Source: CAD feature listing. Evaluate the final solid. Frame: model axes, mm. A direction names the side the tool comes from. Coordinates: 2 decimals unless noted, no trailing zeros. Loops run counter-clockwise (first coordinate to the right, second up) from the corner with the lowest first, then second, coordinate; pieces in that order, holes last. Notation, with made-up numbers: (-12, 2) - (-5, 2) arc R21 ccw to (-5, 16) - close; hole circle Ø8 at (27.5, 67.25). An arc over 180 degrees is marked (long way). Use CSV: the item, a comma, the result in double quotes. Start each with the question number.
Autodesk Inventor part; units mm, degrees
ref_plane "YZ Plane" through (0, 0, 0) normal (1, 0, 0) x (0, 1, 0)
ref_plane "XZ Plane" through (0, 0, 0) normal (0, 1, 0) x (-1, 0, 0)
ref_plane "XY Plane" through (0, 0, 0) normal (0, 0, 1) x (1, 0, 0)
sketch "Sketch1" plane through (0, 0, 0) normal (0, 0, 1) x (1, 0, 0)
  line L0 (-50, 10) -> (50, 10)
  line L1 (50, 10) -> (50, -10)
  line L2 (50, -10) -> (-50, -10)
  line L3 (-50, -10) -> (-50, 10)
  line L4 (-50, 10) -> (50, -10) construction
  line L5 (50, 10) -> (-50, -10) construction
  line L6 (51, 11) -> (-51, 11)
  line L7 (-51, 11) -> (-51, -11)
  line L8 (-51, -11) -> (51, -11)
  line L9 (51, -11) -> (51, 11)
  line L10 (-48, -8) -> (48, -8)
  line L11 (48, -8) -> (48, 8)
  line L12 (48, 8) -> (-48, 8)
  line L13 (-48, 8) -> (-48, -8)
  line L14 (-48, -8) -> (48, 8) construction
  line L15 (48, -8) -> (-48, 8) construction
  line L16 (-48, 0) -> (48, 0) construction
  circle A0 centre (-36, 0) radius 0.5
  circle A1 centre (-12, 0) radius 0.5
  circle A2 centre (12, 0) radius 0.5
  circle A3 centre (36, 0) radius 0.5
  point P0 (0, 0)
  dimension "d0" = 100
  dimension "d1" = 20
  dimension "d2" = 1
  dimension "d7" = 96
  dimension "d8" = 16
  dimension "d9" = 2
  dimension "d10" = 1
  dimension "d11" = 12
  dimension "d12" = 1
  dimension "d13" = 24
  dimension "d14" = 1
  dimension "d15" = 24
  dimension "d16" = 1
  dimension "d17" = 24
extrude "Extrusion3" add sketch "Sketch1" along normal blind 9 contours L9 L8 L7 L6
extrude "Extrusion4" add sketch "Sketch1" along normal blind 1 contours L0 L1 L2 L3
extrude "Extrusion5" add sketch "Sketch1" along normal blind 4 contours L13 L12 L11 L10 | A0 | A1 | A2 | A3
extrude "Extrusion6" cut sketch "Sketch1" along normal blind 4 contours A0 | A1 | A2 | A3
sketch "Sketch2" plane through (-51, -11, 0) normal (0, -1, 0) x (1, 0, 0)
  line L0 (0, 0) -> (0, 9) construction
  line L1 (0, 6.5) -> (102, 6.5) construction
  line L2 (102, 0) -> (102, 9) construction
  line L3 (0, 0) -> (102, 0) construction
  circle A0 centre (15, 6.5) radius 0.5
  circle A1 centre (39, 6.5) radius 0.5
  circle A2 centre (63, 6.5) radius 0.5
  circle A3 centre (87, 6.5) radius 0.5
  point P0 (51, 0)
  dimension "d26" = 6.5
  dimension "d27" = 1
  dimension "d28" = 15
  dimension "d29" = 1
  dimension "d30" = 24
  dimension "d31" = 1
  dimension "d32" = 24
  dimension "d33" = 1
  dimension "d34" = 24
extrude "Extrusion7" cut sketch "Sketch2" against normal blind 2
sketch "Sketch3" plane through (-36, -11, 0) normal (-1, 0, 0) x (0, 0, 1)
  line L0 (11.6401, 26.0282) -> (-2.7437, 26.0282)
  line L1 (-2.7437, 26.0282) -> (-2.7437, -4.1114)
  line L2 (-2.7437, -4.1114) -> (11.6401, -4.1114)
  line L3 (11.6401, -4.1114) -> (11.6401, 26.0282)
  point P0 (0, 11)
properties part number "eit_chamber_electrode_side"
(1) Ray query, line 1 (Y direction, x = 5, z = 1.5); line 2 (X direction, y = -2.75, z = 3.25); line 3 (Y direction, x = -36, z = 2.2). Return the intervals inside material, ascending. Write a range as [from, to].
(2) Section C-C on y = -9. Output: boundary loops of the cut face in (x, z), plus the area to 3 significant figures.
(3) Section B-B on x = -17.5. Output: boundary loops of the cut face in (y, z), plus the area to 3 significant figures.
(4) Pin query (flat end, axial travel): pin 1 Ø1 at (x, y) = (-9.5, -7.5) entering from +Z. Return the tip coordinate at first contact, or that it passes through.
(5) Section A-A on y = -4.5. Output: boundary loops of the cut face in (x, z), plus the area to 3 significant figures.
(6) Draft query along X for faces 3 (the flat face through (51, 0, 4)), 4 (the flat face through (50, 0, 5)), 5 (the flat face through (-1, 0, 0)). Return one class per face: released by +X, released by -X, zero draft, split by the parting line, or undercut.
(7) Reachability of faces 1 (the flat face through (1, 8, 2)), 2 (the flat face through (-0.2, 10.6, 9)) from +Z, -Z, +X, -X, +Y, -Y: full face, straight path, thin tool, end or side. Return the list, or none.
Solution:
1,line 1,"y = [-11, -10], [-8, 8], [10, 11]"
1,line 2,"x = [-51, -50], [-48, 48], [50, 51]"
1,line 3,"y = [-11, -10], [-8, -0.5], [0.5, 8], [10, 11]"
2,outline,"(-51, 0) - (51, 0) - (51, 9) - (50, 9) - (50, 1) - (-50, 1) - (-50, 9) - (-51, 9) - close"
2,area,"118 mm²"
3,outline,"(-11, 0) - (11, 0) - (11, 9) - (10, 9) - (10, 1) - (8, 1) - (8, 4) - (-8, 4) - (-8, 1) - (-10, 1) - (-10, 9) - (-11, 9) - close"
3,area,"86.0 mm²"
4,pin 1,"stops at z = 4"
5,outline,"(-51, 0) - (51, 0) - (51, 9) - (50, 9) - (50, 1) - (48, 1) - (48, 4) - (-48, 4) - (-48, 1) - (-50, 1) - (-50, 9) - (-51, 9) - close"
5,area,"406 mm²"
6,face 3,"released by +X"
6,face 4,"undercut"
6,face 5,"zero draft"
7,face 1,"+Z"
7,face 2,"+Z, +X, -X, +Y, -Y"
